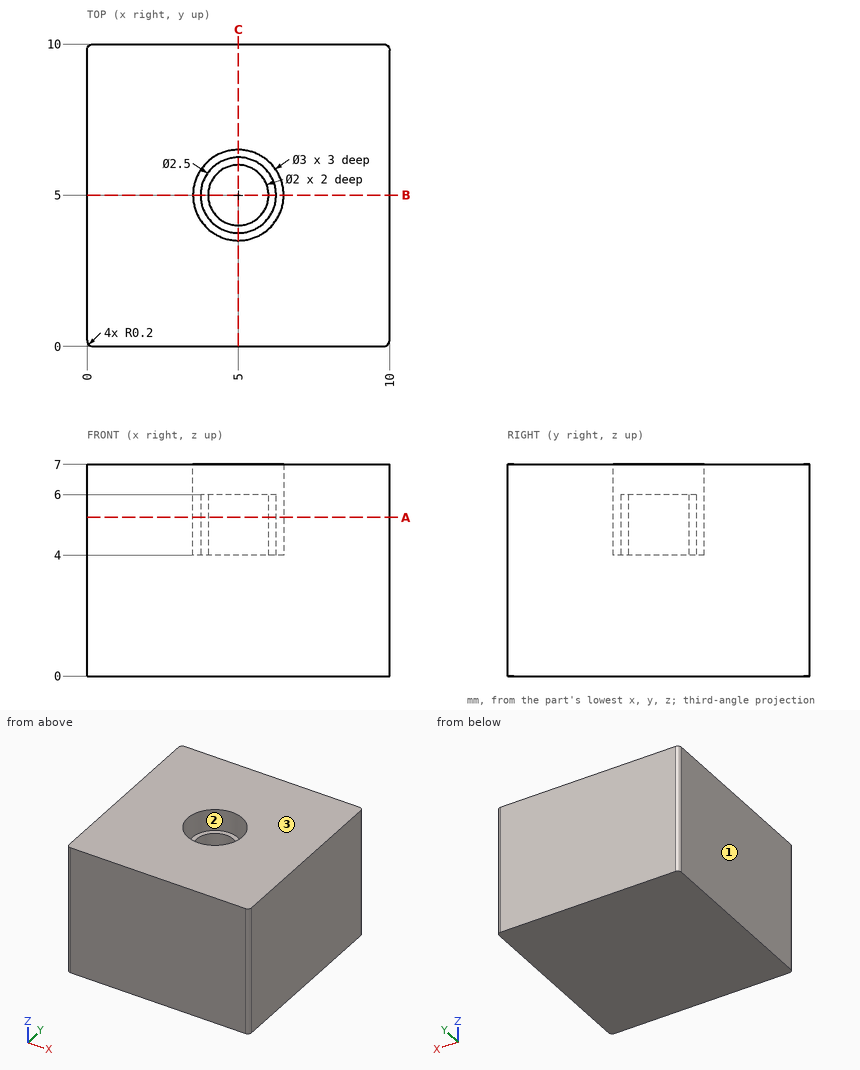
Drawing for the job (mm, zero at the part's lowest x, y, z). Round coordinates to 2 decimals unless told otherwise and drop trailing zeros. Order: outer loops, then holes, each group sorted by start corner. A loop starts at its lowest first (then second) coordinate and runs counter-clockwise, first axis right, second up. Notation, with made-up numbers: (-37, 2) -> (16, 2) arc R8 cw to (16, 11) -> close; hole circle Ø8 at (-0.75, 23). An arc over 180 degrees is marked (long way). Put each result on its own line as item: value.
Q1. Wall check: line 1 (Y direction, x = 5, z = 5.2); line 2 (Y direction, x = 5, z = 6.3). Give the ranges that are in metal, low to high. Write a range as [from, to].
From the geometry:
line 1: y = [0, 3.5], [3.75, 4], [6, 6.25], [6.5, 10]
line 2: y = [0, 3.5], [6.5, 10]
Q2. Band-saw the part on A-A (z = 5.25). Give the cut face in (x, y), and give its area (3 significant figures).
From the geometry:
outline: (0, 0.2) arc R0.2 ccw to (0.2, 0) -> (9.8, 0) arc R0.2 ccw to (10, 0.2) -> (10, 9.8) arc R0.2 ccw to (9.8, 10) -> (0.2, 10) arc R0.2 ccw to (0, 9.8) -> close; circle Ø2.5 at (5, 5); hole circle Ø3 at (5, 5); hole circle Ø2 at (5, 5)
area: 94.7 mm2
Q3. Pin check, flat tips, straight feed: pin 1 Ø1.6 at (x, y) = (4.5, 5) entering from +Z; pin 2 Ø0.8 at (x, y) = (5, 5.5) entering from +Z. Stop position of each tip, or through.
From the geometry:
pin 1: stops at z = 6
pin 2: stops at z = 4
Q4. Pull direction X, two halves, no side cores. Call the marked faces 1, 2 and 3: pulls with the +X half, pulls with the -X half, needs draft (parallel to the pull), parting line crosses it, or undercut.
From the geometry:
face 1: pulls with the -X half
face 2: undercut
face 3: needs draft
Q5. Band-saw the part on B-B (y = 5). Give the cut face in (x, z), and give its area (3 significant figures).
From the geometry:
outline: (0, 0) -> (10, 0) -> (10, 7) -> (6.5, 7) -> (6.5, 4) -> (6.25, 4) -> (6.25, 6) -> (6, 6) -> (6, 4) -> (4, 4) -> (4, 6) -> (3.75, 6) -> (3.75, 4) -> (3.5, 4) -> (3.5, 7) -> (0, 7) -> close
area: 62.0 mm2
